from build123d import *

# Parameters (mm, degrees)
F0_W     = 254
F0_H     = 273.05
F0_R     = 1.6
F0_R_2   = 2.1
F1_DEPTH = 4.7625
F2_W     = 25.4
F2_H     = 4.7625
F2_W_2   = 4.7625
F2_H_2   = 25.4
F3_DEPTH = 25.4


with BuildPart() as f1:
    # F0 (on Top) → F1 (new body)
    with BuildSketch(Plane.XY):
        with Locations((127, 136.525)):
            Rectangle(F0_W, F0_H)
        with Locations((21, 11.2625)):
            Circle(F0_R, mode=Mode.SUBTRACT)
        with Locations((21, 43.2625)):
            Circle(F0_R, mode=Mode.SUBTRACT)
        with Locations((21, 56.025)):
            Circle(F0_R, mode=Mode.SUBTRACT)
        with Locations((21, 88.025)):
            Circle(F0_R, mode=Mode.SUBTRACT)
        with Locations((21, 100.7875)):
            Circle(F0_R, mode=Mode.SUBTRACT)
        with Locations((21, 132.7875)):
            Circle(F0_R, mode=Mode.SUBTRACT)
        with Locations((233, 11.2625)):
            Circle(F0_R, mode=Mode.SUBTRACT)
        with Locations((233, 43.2625)):
            Circle(F0_R, mode=Mode.SUBTRACT)
        with Locations((233, 56.025)):
            Circle(F0_R, mode=Mode.SUBTRACT)
        with Locations((233, 88.025)):
            Circle(F0_R, mode=Mode.SUBTRACT)
        with Locations((233, 100.7875)):
            Circle(F0_R, mode=Mode.SUBTRACT)
        with Locations((233, 132.7875)):
            Circle(F0_R, mode=Mode.SUBTRACT)
        with Locations((43.6125, 179.4475)):
            Circle(F0_R_2, mode=Mode.SUBTRACT)
        with Locations((43.6125, 229.4475)):
            Circle(F0_R_2, mode=Mode.SUBTRACT)
        with Locations((193.6125, 179.4475)):
            Circle(F0_R_2, mode=Mode.SUBTRACT)
        with Locations((193.6125, 229.4475)):
            Circle(F0_R_2, mode=Mode.SUBTRACT)
    extrude(amount=F1_DEPTH)

    # F2 (on face) → F3 (cut)
    with BuildSketch(Plane.XY.offset(4.7625)):
        with Locations((38.1, 2.38125)):
            Rectangle(F2_W, F2_H)
        with Locations((88.9, 2.38125)):
            Rectangle(F2_W, F2_H)
        with Locations((139.7, 2.38125)):
            Rectangle(F2_W, F2_H)
        with Locations((190.5, 2.38125)):
            Rectangle(F2_W, F2_H)
        with Locations((241.3, 2.38125)):
            Rectangle(F2_W, F2_H)
        with Locations((2.38125, 241.3)):
            Rectangle(F2_W_2, F2_H_2)
        with Locations((2.38125, 190.5)):
            Rectangle(F2_W_2, F2_H_2)
        with Locations((2.38125, 139.7)):
            Rectangle(F2_W_2, F2_H_2)
        with Locations((2.38125, 88.9)):
            Rectangle(F2_W_2, F2_H_2)
        with Locations((2.38125, 38.1)):
            Rectangle(F2_W_2, F2_H_2)
        with Locations((251.61875, 241.3)):
            Rectangle(F2_W_2, F2_H_2)
        with Locations((251.61875, 190.5)):
            Rectangle(F2_W_2, F2_H_2)
        with Locations((251.61875, 139.7)):
            Rectangle(F2_W_2, F2_H_2)
        with Locations((251.61875, 88.9)):
            Rectangle(F2_W_2, F2_H_2)
        with Locations((251.61875, 38.1)):
            Rectangle(F2_W_2, F2_H_2)
        with Locations((38.1, 270.66875)):
            Rectangle(F2_W, F2_H)
        with Locations((88.9, 270.66875)):
            Rectangle(F2_W, F2_H)
        with Locations((139.7, 270.66875)):
            Rectangle(F2_W, F2_H)
        with Locations((190.5, 270.66875)):
            Rectangle(F2_W, F2_H)
        with Locations((241.3, 270.66875)):
            Rectangle(F2_W, F2_H)
    extrude(amount=-F3_DEPTH, mode=Mode.SUBTRACT)


solid = f1.part
The listing builds one solid part. Answer for the finished solid, in the listing's coordinates (mm). Give positions to 0.01 mm unless a question says otherwise; leave off trailing zeros. Loops run counter-clockwise (first coordinate to the right, second up) from the corner with the lowest first, then second, coordinate; pieces in that order, holes last. Notation, with made-up numbers: (52, 50) - (68, 50) arc R29 ccw to (68, 72) - close; hole circle Ø1 at (-31, 37). An arc over 180 degrees is marked (long way). Answer as a JSON object with one key per item and string values.
1. A cutting plane is placed at C-C (z = 1.8). Give the number of separate pieces and of enclosed holes in the cut face, then the cut area to 3 significant figures.
Determined:
{"separate pieces": "1", "enclosed holes": "16", "area": "66,800 mm²"}
2. Find the intervals of material crossed by L1, parallel to X at y = 44, z = 2; L2, parallel to Y at x = 241.5, z = 3.05; L3, parallel to X at y = 197.5, z = 3.35, in increasing order. Write a range as [from, to].
Determined:
{"L1": "[4.76, 19.58], [22.42, 231.58], [234.42, 249.24]", "L2": "[4.76, 268.29]", "L3": "[4.76, 249.24]"}
3. Flat-ended cylindrical pins translate along their axes: pin 1 Ø1.9 at (x, y) = (233, 11.26) entering from +Z; pin 2 Ø1.4 at (x, z) = (247.5, 1.5) entering from -Y. Find the tip coordinate at first contact, or state that the pin passes through.
Determined:
{"pin 1": "through", "pin 2": "y = 4.76"}
4. A cutting plane is placed at A-A (x = 85). Write down the section's boundary in (y, z), then the cut area to 3 significant figures.
Determined:
{"outline": "(4.76, 0) - (268.29, 0) - (268.29, 4.76) - (4.76, 4.76) - close", "area": "1,260 mm²"}
5. A cutting plane is placed at B-B (y = 187.5). Write down the section's boundary in (x, z), then the cut area to 3 significant figures.
Determined:
{"outline": "(4.76, 0) - (249.24, 0) - (249.24, 4.76) - (4.76, 4.76) - close", "area": "1,160 mm²"}
